Solid Edge part; units mm, degrees
sketch "Sketch1" plane through (0, 0, 0) normal (0, 0, 1) x (1, 0, 0)
  circle A0 centre (0, 0) radius 4
extrude "Protrusion1" add sketch "Sketch1" along normal blind 47.5
hole "Hole_3" at (0, 0, 0) direction (0, 0, 1) diameter 3.242 depth 10 thread major 4 thread length 8
hole "Hole_4" at (0, 0, 47.5) direction (0, 0, -1) diameter 3.242 depth 10 thread major 4 thread length 8
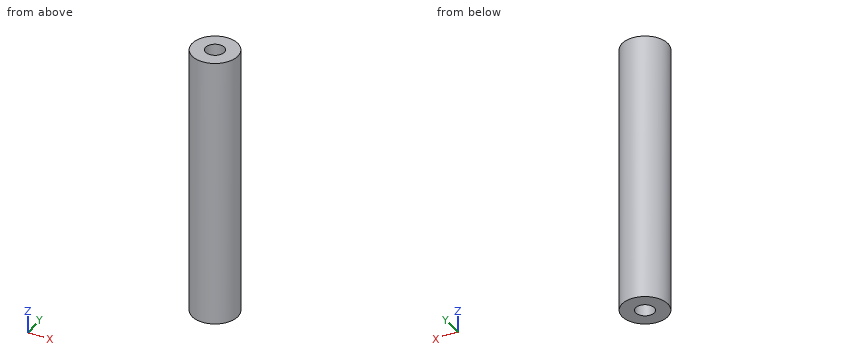
Input: part model. Units: mm. Frame: model coordinates. Give positions to 0.01 mm unless a question says otherwise; leave off trailing zeros. Write each loop counter-clockwise with the first axis right and the second up, starting at its lowest first coordinate (ties: lowest second). Pieces come first, ordered by that corner, then holes. Notation, with made-up numbers: (-0.5, -12.75) - (52.5, -12.75) arc R32 cw to (52.5, 17.25) - close; hole circle Ø9 at (59, 9.25). An arc over 180 degrees is marked (long way). Write item = value, one per line. Start each with the question number.
1) Cut plane D-D (z = 32). Return loops of the section in (x, y), and give its area (3 significant figures).
2) Material intervals for L1, parallel to Y at x = 0, z = 45; L2, parallel to X at y = -1.25, z = 44; L3, parallel to X at y = 0.25, z = 24, sorted ascending. Write a range as [from, to].
3) Pin query (flat end, axial travel): pin 1 (1 mm diameter, centred on x = 0.5, y = -0.5, fed in from +Z); pin 2 (2.5 mm diameter, centred on x = 0, y = 0, fed in from -Z). Return the tip coordinate at first contact, or that it passes through.
4) Cut plane A-A (y = 0). Return loops of the section in (x, z), and give its area (3 significant figures).
5) Cut plane B-B (z = 4). Return loops of the section in (x, y), and give its area (3 significant figures).
Answers follow:
q1.outline = circle Ø8 at (0, 0)
q1.area = 50.3 mm^2
q2.L1 = [-4, -1.62], [1.62, 4]
q2.L2 = [-3.8, -1.03], [1.03, 3.8]
q2.L3 = [-3.99, 3.99]
q3.pin_1 = 37.5
q3.pin_2 = 10
q4.outline = (-4, 0) - (-1.62, 0) - (-1.62, 10) - (1.62, 10) - (1.62, 0) - (4, 0) - (4, 47.5) - (1.62, 47.5) - (1.62, 37.5) - (-1.62, 37.5) - (-1.62, 47.5) - (-4, 47.5) - close
q4.area = 315 mm^2
q5.outline = circle Ø8 at (0, 0); hole circle Ø3.24 at (0, 0)
q5.area = 42.0 mm^2
